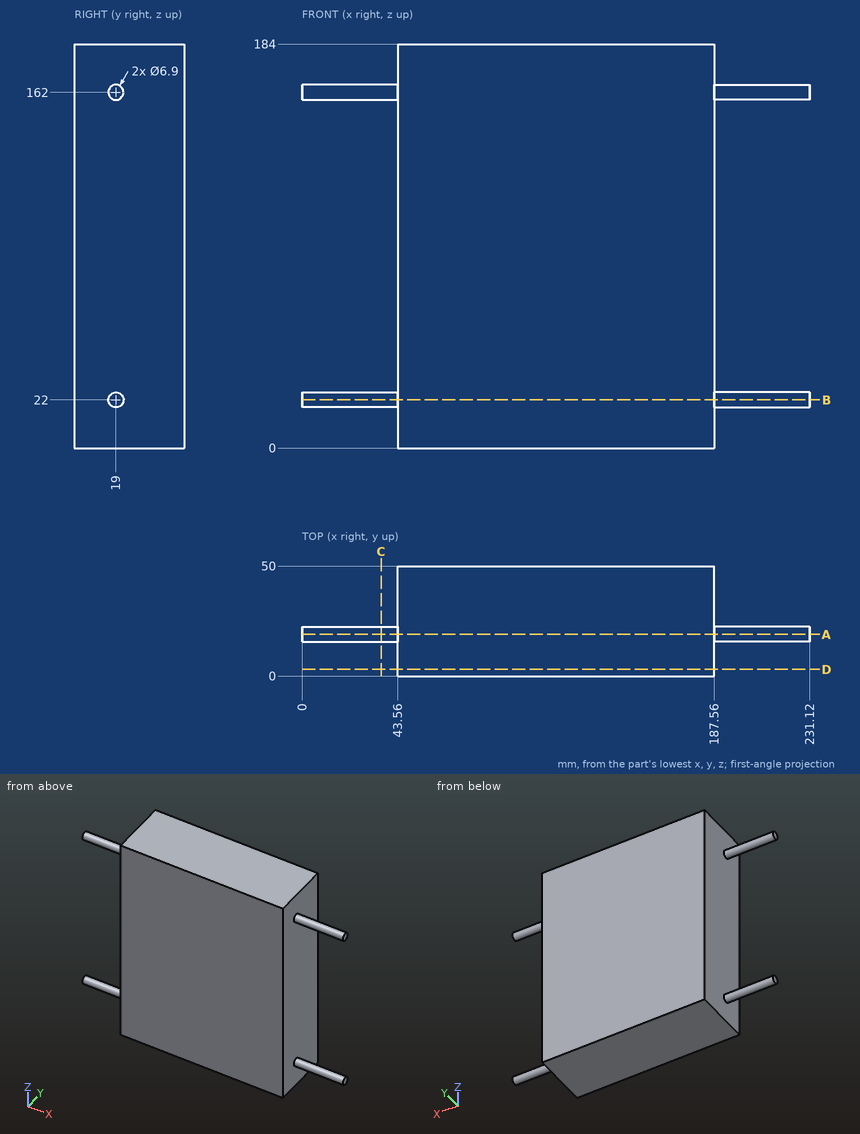
For this review, use the dimensioned drawing (mm, ordinates from the lowest corner) and the shaded views. Coordinates: 2 decimals unless noted, no trailing zeros. Loops run counter-clockwise (first coordinate to the right, second up) from the corner with the lowest first, then second, coordinate; pieces in that order, holes last. Notation, with made-up numbers: (13, -36) -> (48, -36) arc R29 cw to (48, -16) -> close; hole circle Ø3 at (-34, 32). An arc over 180 degrees is marked (long way). Write each question's results on one line, items separated by ' | '.
Q1. For pin 1 Ø25 at (y, z) = (25.5, 89.5) entering from -X; pin 2 Ø25 at (y, z) = (30.5, 131) entering from +X; pin 3 Ø2 at (x, z) = (29.5, 161.5) entering from +Y, all flat-tipped, find the tip position at first contact; note any pin that passes through.
Taken from the geometry:
pin 1: x = 43.56 | pin 2: x = 187.56 | pin 3: y = 22.45
Q2. Add section C-C, the plane x = 36. State the section outline as (y, z) points.
Taken from the geometry:
outline: circle Ø6.9 at (19, 22); circle Ø6.9 at (19, 162)
Q3. Add section A-A, the plane y = 19. State the section outline as (x, z) points.
Taken from the geometry:
outline: (0, 18.55) -> (43.56, 18.55) -> (43.56, 0) -> (187.56, 0) -> (187.56, 18.55) -> (231.12, 18.55) -> (231.12, 25.45) -> (187.56, 25.45) -> (187.56, 158.55) -> (231.12, 158.55) -> (231.12, 165.45) -> (187.56, 165.45) -> (187.56, 184) -> (43.56, 184) -> (43.56, 165.45) -> (0, 165.45) -> (0, 158.55) -> (43.56, 158.55) -> (43.56, 25.45) -> (0, 25.45) -> close
Q4. Add section D-D, the plane y = 3. State the section outline as (x, z) points.
Taken from the geometry:
outline: (43.56, 0) -> (187.56, 0) -> (187.56, 184) -> (43.56, 184) -> close
Q5. Add section B-B, the plane z = 22. State the section outline as (x, y) points, then the cut area to 3 significant figures.
Taken from the geometry:
outline: (0, 15.55) -> (43.56, 15.55) -> (43.56, 0) -> (187.56, 0) -> (187.56, 15.55) -> (231.12, 15.55) -> (231.12, 22.45) -> (187.56, 22.45) -> (187.56, 50) -> (43.56, 50) -> (43.56, 22.45) -> (0, 22.45) -> close | area: 7,800 mm²
Q6. To check wall thickness, follow line 1 along Z through (x, y) = (31.5, 19); line 2 along X through (y, z) = (38, 158.5); line 3 along Z through (x, y) = (191, 22). State the ranges of each line that lie inside material, in increasing order. Write a range as [from, to].
Taken from the geometry:
line 1: [18.55, 25.45], [158.55, 165.45] | line 2: [43.56, 187.56] | line 3: [20.3, 23.7], [160.3, 163.7]
